The model under review builds one solid part; all positions refer to its coordinate system, in mm. Give positions to 0.01 mm unless a question says otherwise; leave off trailing zeros. Write each loop counter-clockwise with the first axis right and the second up, starting at its lowest first coordinate (ties: lowest second). Pieces come first, ordered by that corner, then holes. Notation, with made-up numbers: (56, 85) - (60, 85) arc R30 ccw to (60, 121) - close; hole circle Ø10 at (25, 36.25). An arc over 180 degrees is marked (long way). One line per question, with ' | ' between items. Start each with the question number.
```python
from build123d import *

# Parameters (mm, degrees)
SKETCH_1_W                   = 80
SKETCH_1_H                   = 20
EXTRUDE_1_DEPTH              = 3
HOLE_WIZARD_M2_1_D           = 1.6
HOLE_WIZARD_M2_1_CSINK_D     = 2.05
HOLE_WIZARD_M2_1_CSINK_ANGLE = 90


with BuildPart() as part:
    # 草图1 → 凸台-拉伸1 (new body)
    with BuildSketch(Plane(origin=(0, 0, 0), x_dir=(1, 0, 0), z_dir=(0, 1, 0))):
        with Locations((40, 10)):
            Rectangle(SKETCH_1_W, SKETCH_1_H)
    extrude(amount=EXTRUDE_1_DEPTH)

    # M2 螺纹孔1 (through all)
    with Locations(Plane(origin=(0, 3, 0), x_dir=(1, 0, 0), z_dir=(0, 1, 0))):
        with Locations((8.5, 15), (11.2, 5), (71.5, 15), (68.8, 5)):
            CounterSinkHole(HOLE_WIZARD_M2_1_D / 2, HOLE_WIZARD_M2_1_CSINK_D / 2, counter_sink_angle=HOLE_WIZARD_M2_1_CSINK_ANGLE)


solid = part.part
```
Item 1: Take a section at A-A (z = -15). Give the boundary of the cut face in (x, y) (3 decimals).
Item 2: The part is to be moulded in two halves that separate along Z. For faces 1 (the cylindrical face through (12, 1, -5)), 2 (the flat face through (39, 1, 0)), 3 (the flat face through (39, 1, -20)), 4 (the flat face through (39, 0, -10)), say which applies: +Z half, -Z half, draft (parallel to the pull), parting line (faces both ways), or undercut.
Item 3: Clearance check with flat-ended pins moving along their axes: P1, Ø1.3, axis at x = 11.2, z = -5, coming from the -Y side; P2, Ø1.8, axis at x = 71.5, z = -15, coming from the +Y side (3 decimals). State where each tip first meets the part, or that it passes through.
Item 4: Take a section at B-B (x = 8.5). Give the boundary of the cut face in (y, z) (3 decimals), plus the area to 3 significant figures.
Item 5: For probe 1 along X at (y, z) = (1.4, -5); probe 2 along X at (y, z) = (2.05, -15); probe 3 along Z at (x, y) = (71.5, 2.1), list the stretches that pass through material, from the lowest coordinate up.
Check sheet entries:
1) outline: (0, 0) - (7.7, 0) - (7.7, 2.775) - (7.475, 3) - (0, 3) - close; (9.3, 0) - (70.7, 0) - (70.7, 2.775) - (70.475, 3) - (9.525, 3) - (9.3, 2.775) - close; (72.3, 0) - (80, 0) - (80, 3) - (72.525, 3) - (72.3, 2.775) - close
2) face 1: undercut | face 2: +Z half | face 3: -Z half | face 4: draft
3) P1: passes through | P2: stops at y = 2.875
4) outline: (0, -20) - (3, -20) - (3, -16.025) - (2.775, -15.8) - (0, -15.8) - close; (0, -14.2) - (2.775, -14.2) - (3, -13.975) - (3, 0) - (0, 0) - close | area: 55.1 mm^2
5) probe 1: x = 0 to 10.4, 12 to 68, 69.6 to 80 | probe 2: x = 0 to 7.7, 9.3 to 70.7, 72.3 to 80 | probe 3: z = -20 to -15.8, -14.2 to 0
